Geometry check sheet. Reference: the model listing, model coordinates, mm. Round coordinates to 2 decimals unless told otherwise and drop trailing zeros. Write each loop counter-clockwise with the first axis right and the second up, starting at its lowest first coordinate (ties: lowest second). Pieces come first, ordered by that corner, then holes. Notation, with made-up numbers: M 36,-21 L 82,-21 A21 cw 82,-13 Z; hole C 62.5,38 d1. An arc over 180 degrees is marked long. Use a Markdown table: item, result.
```python
from build123d import *


with BuildPart() as part:
    # Sketch1 → Revolve1 (revolve)
    with BuildSketch(Plane.XY):
        with BuildLine():
            Line((-28.5, 60), (-26, 60))
            Line((-26, 60), (-22, 64))
            Line((-22, 64), (-16, 64))
            Line((-16, 64), (-16, 56))
            Line((-16, 56), (-18.790689802, 56))
            ThreePointArc((-18.790689802, 56), (-34.407796248, 29.913629212), (-39.845400687, 0))
            Line((-39.845400687, 0), (-49.845400687, 0))
            ThreePointArc((-49.845400687, 0), (-44.350112671, 31.841899011), (-28.5, 60))
        make_face()
    revolve(axis=Axis((-162.413763562, 0, 0), (1, 0, 0)))


solid = part.part
```
Item 1: Material ranges on line 1 along Z through (x, y) = (-17, 0); line 2 along Y through (x, z) = (-17, 24.5); line 3 along X through (y, z) = (0, -1), recorded low to high. Write a range as from..to.
Outcome:
| item | result |
|---|---|
| line 1 | z = -64..-56, 56..64 |
| line 2 | y = -59.12..-50.36, 50.36..59.12 |
| line 3 | x = -49.84..-39.84 |
Item 2: Mould release check, pull along Y, two halves, no side actions. Record for faces 1 (the face through (-27.23, -59.94, 2.64)), 2 (the face through (-16, 0, -57)), 3 (the face through (-17.41, 51.73, -21.45)): +Y half, -Y half, draft (parallel to the pull), parting line (faces both ways), or undercut.
Outcome:
| item | result |
|---|---|
| face 1 | parting line |
| face 2 | draft |
| face 3 | undercut |
Item 3: Go/stop test with flat-tipped pins: pin 1 (3 mm diameter, centred on y = 31.5, z = -38.5, fed in from +X); pin 2 (12 mm diameter, centred on x = -40, z = -24, fed in from -Y); pin 3 (4 mm diameter, centred on y = -40.5, z = -50, fed in from -X). Record where each tip stops, or that it passes through.
Outcome:
| item | result |
|---|---|
| pin 1 | stops at x = -22.66 |
| pin 2 | stops at y = -47.15 |
| pin 3 | stops at x = -23.66 |
Item 4: Cross-section at A-A, the plane y = 0. Record the cut outline in (x, z).
Outcome:
| item | result |
|---|---|
| outline | M -28.5,-60 L -26,-60 L -22,-64 L -16,-64 L -16,-56 L -18.79,-56 A85 cw -18.79,56 L -16,56 L -16,64 L -22,64 L -26,60 L -28.5,60 A95 ccw Z |
